Design review of the part shown in the three views and the two pictorial views. Dimensions are in mm from the part's minimum x, y and z. A direction names the side the tool comes from. Round coordinates to 2 decimals unless told otherwise and drop trailing zeros. Order: outer loops, then holes, each group sorted by start corner. A loop starts at its lowest first (then second) coordinate and runs counter-clockwise, first axis right, second up. Notation, with made-up numbers: (-25.75, -1) - (24.25, -1) arc R34 cw to (24.25, 36) - close; hole circle Ø4 at (79.5, 69.5). An arc over 180 degrees is marked (long way). Use CSV: the item, a comma, the result in double quotes.
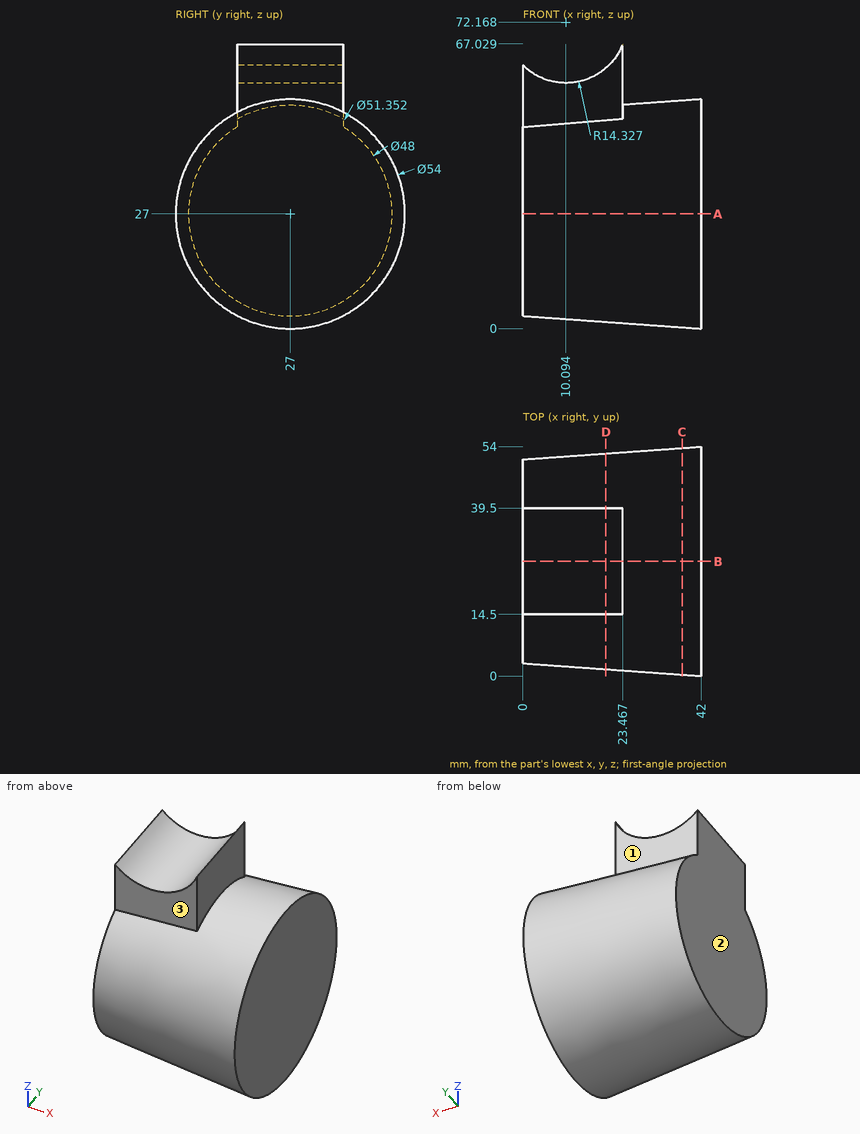
1) To check wall thickness, follow L1, parallel to Z at x = 34, y = 48 (1 decimal); L2, parallel to Z at x = 5, y = 42; L3, parallel to Y at x = 4.5, z = 41. State the ranges of each line that lie inside material, in increasing order. Write a range as from..to.
Data:
L1,"z = 11..43"
L2,"z = 7.81..46.19"
L3,"y = 7.11..46.89"
2) Insertion check: pin 1 Ø6 at (x, z) = (9.5, 54.5) entering from +Y; pin 2 Ø2 at (x, y) = (22, 47) entering from +Z; pin 3 Ø15.5 at (x, z) = (6, 59) entering from -Y. Each pin has a flat end and moves straight along its axis. Give the tip position at first contact, or say it passes through.
Data:
pin 1,"stops at y = 39.5"
pin 2,"stops at z = 44.12"
pin 3,"stops at y = 14.5"
3) For the marked faces 1, 2 and 3, list the 3-axis set-ups (+Z, -Z, +X, -X, +Y, -Y) from which the entire face can be reached by the end or side of a thin tool; tool diameter is ignored.
Data:
face 1,"+Z, -X, +Y"
face 2,"+Z, -Z, -X, +Y, -Y"
face 3,"+Z, -X, -Y"
4) We need section C-C (x = 37.5). Give the boundary of the cut face in (y, z).
Data:
outline,"circle Ø53.36 at (27, 27)"
5) We need section A-A (z = 27). Give the boundary of the cut face in (x, y).
Data:
outline,"(0, 3) - (42, 0) - (42, 54) - (0, 51) - close"
6) We need section B-B (y = 27). Give the boundary of the cut face in (x, z), then the cut area to 3 significant figures.
Data:
outline,"(0, 3) - (42, 0) - (42, 54) - (23.47, 52.68) - (23.47, 67.03) arc R14.33 cw to (0, 62) - close"
area,"2,330 mm2"
7) We need section D-D (x = 19.5). Give the boundary of the cut face in (y, z) (1 decimal), then the cut area to 3 significant figures.
Data:
outline,"(14.5, 49.1) arc R25.4 ccw (long way) to (39.5, 49.1) - (39.5, 61.4) - (14.5, 61.4) - close"
area,"2,280 mm2"
